Check sheet for the modelled part. Datum: model origin and axes. Units: mm. Round coordinates to 2 decimals unless told otherwise and drop trailing zeros. Order: outer loops, then holes, each group sorted by start corner. A loop starts at its lowest first (then second) coordinate and runs counter-clockwise, first axis right, second up. Notation, with made-up numbers: M -6,-11 L 17,-11 A31 ccw 17,27 Z; hole C 83,-39 d10. An arc over 180 degrees is marked long. One line per item, written item: value. Start each with the question number.
(1) Thickness scan on L1, parallel to X at y = 8, z = 0.45; L2, parallel to Y at x = -39, z = 1.25; L3, parallel to X at y = 14, z = 1.25. Record the ranges inside material, lowest first.
(2) Cross-section at C-C, the plane x = -38.5. Enter the section's corners in (y, z).
(3) Cross-section at B-B, the plane y = 13. Enter the section's corners in (x, z).
(4) Cross-section at A-A, the plane z = 1.2. Enter the section's corners in (x, y), and give its area (3 significant figures).
(5) Cross-section at D-D, the plane y = 6.5. Enter the section's corners in (x, z).
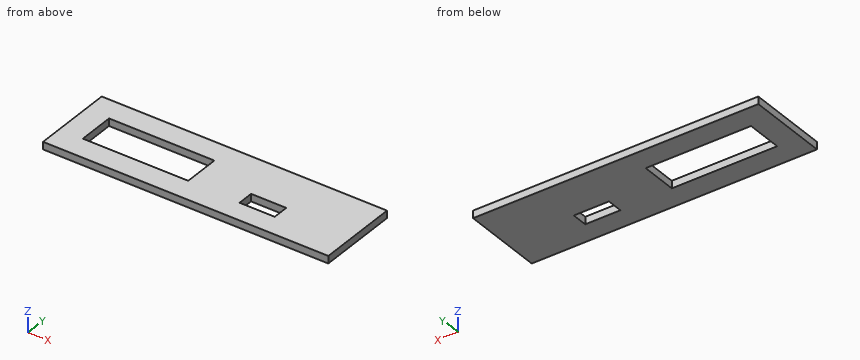
from build123d import *

# Parameters (mm, degrees)
F0_W     = 68.78
F0_H     = 19.67
F1_DEPTH = 1.78
F2_W     = 25.4
F2_H     = 8.776869
F3_DEPTH = 25.4
F4_W     = 8.480195
F4_H     = 3.840108
F5_DEPTH = 1.781


with BuildPart() as f1:
    # F0 (on Top) → F1 (new body)
    with BuildSketch(Plane.XY):
        with Locations((-34.39, 9.835)):
            Rectangle(F0_W, F0_H)
    extrude(amount=F1_DEPTH)

    # F2 (on face) → F3 (cut)
    with BuildSketch(Plane.XY.offset(1.78)):
        with Locations((-50.408047, 9.845546)):
            Rectangle(F2_W, F2_H)
    extrude(amount=-F3_DEPTH, mode=Mode.SUBTRACT)

    # F4 (on Top) → F5 (cut, through all)
    with BuildSketch(Plane.XY):
        with Locations((-20.799336, 6.992206)):
            Rectangle(F4_W, F4_H)
    extrude(amount=F5_DEPTH, mode=Mode.SUBTRACT)


solid = f1.part
Values found:
1. L1: -68.78 to -63.11, -37.71 to -25.04, -16.56 to 0
1. L2: 0 to 5.46, 14.23 to 19.67
1. L3: -68.78 to -63.11, -37.71 to 0
2. outline: M 0,0 L 5.46,0 L 5.46,1.78 L 0,1.78 Z; M 14.23,0 L 19.67,0 L 19.67,1.78 L 14.23,1.78 Z
3. outline: M -68.78,0 L -63.11,0 L -63.11,1.78 L -68.78,1.78 Z; M -37.71,0 L 0,0 L 0,1.78 L -37.71,1.78 Z
4. outline: M -68.78,0 L 0,0 L 0,19.67 L -68.78,19.67 Z; hole M -63.11,5.46 L -37.71,5.46 L -37.71,14.23 L -63.11,14.23 Z; hole M -25.04,5.07 L -16.56,5.07 L -16.56,8.91 L -25.04,8.91 Z
4. area: 1,100 mm^2
5. outline: M -68.78,0 L -63.11,0 L -63.11,1.78 L -68.78,1.78 Z; M -37.71,0 L -25.04,0 L -25.04,1.78 L -37.71,1.78 Z; M -16.56,0 L 0,0 L 0,1.78 L -16.56,1.78 Z
